Check sheet for the modelled part. Datum: model origin and axes. Units: mm. A direction names the side the tool comes from. Round coordinates to 2 decimals unless told otherwise and drop trailing zeros. Use one line per item in the form item = value. Start each with the question number.
Autodesk Inventor part; units mm, degrees
ref_plane "YZ Plane" through (0, 0, 0) normal (1, 0, 0) x (0, 1, 0)
ref_plane "XZ Plane" through (0, 0, 0) normal (0, 1, 0) x (-1, 0, 0)
ref_plane "XY Plane" through (0, 0, 0) normal (0, 0, 1) x (1, 0, 0)
sketch "Skizze1" plane through (0, 0, 0) normal (0, 1, 0) x (-1, 0, 0)
  line L0 (77.2474, 30) -> (-16.7526, 30)
  line L1 (-16.7526, 30) -> (-16.7526, -30)
  line L2 (-16.7526, -30) -> (77.2474, -30)
  line L3 (77.2474, -30) -> (77.2474, 30)
  line L4 (-35.5526, 0) -> (96.0474, 0)
  point P0 (0, 0)
  dimension "d0" = 30
  dimension "d1" = 60
  dimension "d2" = 94
extrude "Extrusion1" add sketch "Skizze1" along normal blind 10
sketch "Skizze4" plane through (0, 10, 0) normal (0, 1, 0) x (1, 0, 0)
  circle A0 centre (-14.4974, -15.75) radius 2
  circle A1 centre (-14.4974, 15.75) radius 2
  circle A2 centre (-45.9974, -15.75) radius 2
  circle A3 centre (-45.9974, 15.75) radius 2
  line L0 (35.5526, 0) -> (-96.0474, 0)
  line L1 (16.7526, -30) -> (16.7526, 30)
  line L2 (-77.2474, 30) -> (-77.2474, -30)
  point P0 (0, 0)
  dimension "d21" = 4
  dimension "d22" = 15.75
  dimension "d23" = 15.75
  dimension "d26" = 15.75
  dimension "d27" = 15.75
  dimension "d30" = 4
  dimension "d31" = 4
  dimension "d32" = 4
  dimension "d127" = 31.5
  dimension "d128" = 31.5
  dimension "d129" = 31.25
  dimension "d130" = 31.25
extrude "Extrusion4" cut sketch "Skizze4" against normal blind 10
sketch "Skizze5" plane through (0, 10, 0) normal (0, 1, 0) x (1, 0, 0)
  line L0 (-6.9974, -24) -> (-21.9974, -24)
  line L1 (-21.9974, -24) -> (-21.9974, 24)
  line L2 (-21.9974, 24) -> (-6.9974, 24)
  line L3 (-6.9974, 24) -> (-6.9974, -24)
  line L4 (-38.4974, 24) -> (-53.4974, 24)
  line L5 (-53.4974, 24) -> (-53.4974, -24)
  line L6 (-53.4974, -24) -> (-38.4974, -24)
  line L7 (-38.4974, -24) -> (-38.4974, 24)
  line L8 (35.5526, 0) -> (-96.0474, 0)
  line L9 (16.7526, -30) -> (16.7526, 30)
  line L10 (-77.2474, 30) -> (-77.2474, -30)
  point P0 (0, 0)
  dimension "d35" = 15
  dimension "d36" = 48
  dimension "d37" = 24
  dimension "d38" = 23.75
  dimension "d39" = 15
  dimension "d189" = 16.5
extrude "Extrusion5" cut sketch "Skizze5" against normal blind 1
sketch "Skizze6" plane through (0, 9, 0) normal (0, 1, 0) x (1, 0, 0)
  circle A0 centre (-14.4974, -15.75) radius 3.6
  circle A1 centre (-14.4974, 15.75) radius 3.6
  circle A2 centre (-45.9974, -15.75) radius 3.6
  circle A3 centre (-45.9974, 15.75) radius 3.6
  circle A4 centre (-45.9974, 15.75) radius 2
  circle A5 centre (-45.9974, -15.75) radius 2
  circle A6 centre (-14.4974, 15.75) radius 2
  circle A7 centre (-14.4974, -15.75) radius 2
  circle A8 centre (-3.2474, -15.75) radius 3.6
  circle A9 centre (-3.2474, 15.75) radius 3.6
  circle A10 centre (-45.9974, -15.75) radius 3.6
  circle A11 centre (-53.2474, 15.75) radius 3.6
  circle A12 centre (-53.2474, 15.75) radius 2
  circle A13 centre (-45.9974, -15.75) radius 2
  circle A14 centre (-3.2474, 15.75) radius 2
  circle A15 centre (-3.2474, -15.75) radius 2
  circle A16 centre (-3.2474, -15.75) radius 3.6
  circle A17 centre (-3.2474, 15.75) radius 3.6
  circle A18 centre (-45.9974, -15.75) radius 3.6
  circle A19 centre (-53.2474, 15.75) radius 3.6
  circle A20 centre (-53.2474, 15.75) radius 2
  circle A21 centre (-45.9974, -15.75) radius 2
  circle A22 centre (-3.2474, 15.75) radius 2
  circle A23 centre (-3.2474, -15.75) radius 2
  circle A24 centre (-3.2474, -15.75) radius 3.6
  circle A25 centre (-3.2474, 15.75) radius 3.6
  circle A26 centre (-53.2474, -15.75) radius 3.6
  circle A27 centre (-53.2474, 15.75) radius 3.6
  circle A28 centre (-53.2474, 15.75) radius 2
  circle A29 centre (-53.2474, -15.75) radius 2
  circle A30 centre (-3.2474, 15.75) radius 2
  circle A31 centre (-3.2474, -15.75) radius 2
  line L0 (-77.2474, 30) -> (-77.2474, -30)
  point P0 (0, 0)
  point P1 (0, 0)
  point P2 (0, 0)
  point P3 (0, 0)
  point P4 (-45.7474, 16.7182)
  point P5 (-45.7474, 14.7818)
  point P6 (-45.7474, -14.7818)
  point P7 (-45.7474, -16.7182)
  point P8 (-10.7474, 14.7818)
  point P9 (-10.7474, 16.7182)
  point P10 (-10.7474, -16.7182)
  point P11 (-10.7474, -14.7818)
  dimension "d43" = 7.2
  dimension "d44" = 7.2
  dimension "d45" = 7.2
  dimension "d46" = 7.2
  dimension "d79" = 7.2
  dimension "d80" = 7.2
  dimension "d81" = 7.2
  dimension "d82" = 7.2
  dimension "d83" = 7.2
  dimension "d84" = 7.2
  dimension "d85" = 7.2
  dimension "d86" = 7.2
  dimension "d87" = 7.2
  dimension "d88" = 7.2
  dimension "d89" = 7.2
  dimension "d90" = 7.2
  dimension "d142" = 31.25
  dimension "d143" = 31.25
extrude "Extrusion6" cut sketch "Skizze6" against normal blind 3 contours A0 | A1 | A2 | A3 | A4 | A5 | A6 | A7
sketch "Skizze8" plane through (0, 9, 0) normal (0, 1, 0) x (1, 0, 0)
  circle A0 centre (-14.4974, -5.0565) radius 1.5
  circle A1 centre (-14.4974, 4.9435) radius 1.5
  circle A2 centre (-45.9974, -5.0565) radius 1.5
  circle A3 centre (-45.9974, 4.9435) radius 1.5
  line L0 (-77.2474, 30) -> (-77.2474, -30)
  line L1 (16.7526, -30) -> (16.7526, 30)
  point P0 (0, 0)
  dimension "d56" = 10
  dimension "d57" = 10
  dimension "d58" = 31.25
  dimension "d59" = 31.25
  dimension "d62" = 3
  dimension "d63" = 3
  dimension "d64" = 3
  dimension "d65" = 3
  dimension "d146" = 31.25
extrude "Extrusion7" cut sketch "Skizze8" against normal blind 10
chamfer "Fase1" distance 0.5 angle 45 4 edges at (-47.9974, 6, 15.75) (-47.9974, 6, -15.75) (-16.4974, 6, -15.75) (-16.4974, 6, 15.75)
sketch "Skizze9" plane through (0, 0, 0) normal (0, -1, 0) x (1, 0, 0)
  line L0 (-6.9974, -24) -> (-21.9974, -24)
  line L1 (-21.9974, -24) -> (-21.9974, 24)
  line L2 (-21.9974, 24) -> (-6.9974, 24)
  line L3 (-6.9974, 24) -> (-6.9974, -24)
  line L4 (-38.4974, 24) -> (-53.4974, 24)
  line L5 (-53.4974, 24) -> (-53.4974, -24)
  line L6 (-53.4974, -24) -> (-38.4974, -24)
  line L7 (-38.4974, -24) -> (-38.4974, 24)
  line L8 (34.7526, 0) -> (-91.2474, 0)
  line L9 (16.7526, 30) -> (16.7526, -30)
  line L10 (-77.2474, -30) -> (-77.2474, 30)
  point P0 (0, 0)
  point P1 (0, 0)
  dimension "d71" = 15
  dimension "d72" = 48
  dimension "d73" = 24
  dimension "d75" = 15
  dimension "d144" = 23.75
  dimension "d145" = 23.75
extrude "Extrusion8" cut sketch "Skizze9" against normal blind 1
sketch "Skizze10" plane through (0, 0, 0) normal (0, -1, 0) x (1, 0, 0)
  circle A0 centre (-14.4974, -15.75) radius 3.6
  circle A1 centre (-14.4974, 15.75) radius 3.6
  circle A2 centre (-45.9974, -15.75) radius 3.6
  circle A3 centre (-45.9974, 15.75) radius 3.6
  circle A4 centre (-45.9974, 15.75) radius 2
  circle A5 centre (-45.9974, -15.75) radius 2
  circle A6 centre (-14.4974, 15.75) radius 2
  circle A7 centre (-14.4974, -15.75) radius 2
  circle A8 centre (-3.2474, -15.75) radius 3.6
  circle A9 centre (-3.2474, 15.75) radius 3.6
  circle A10 centre (-45.9974, -15.75) radius 3.6
  circle A11 centre (-53.2474, 15.75) radius 3.6
  circle A12 centre (-53.2474, 15.75) radius 2
  circle A13 centre (-45.9974, -15.75) radius 2
  circle A14 centre (-3.2474, 15.75) radius 2
  circle A15 centre (-3.2474, -15.75) radius 2
  circle A16 centre (-3.2474, -15.75) radius 3.6
  circle A17 centre (-3.2474, 15.75) radius 3.6
  circle A18 centre (-53.2474, -15.75) radius 3.6
  circle A19 centre (-53.2474, 15.75) radius 3.6
  circle A20 centre (-53.2474, 15.75) radius 2
  circle A21 centre (-53.2474, -15.75) radius 2
  circle A22 centre (-3.2474, 15.75) radius 2
  circle A23 centre (-3.2474, -15.75) radius 2
  circle A24 centre (-3.2474, -15.75) radius 3.6
  circle A25 centre (-3.2474, 15.75) radius 3.6
  circle A26 centre (-53.2474, -15.75) radius 3.6
  circle A27 centre (-53.2474, 15.75) radius 3.6
  circle A28 centre (-53.2474, 15.75) radius 2
  circle A29 centre (-53.2474, -15.75) radius 2
  circle A30 centre (-3.2474, 15.75) radius 2
  circle A31 centre (-3.2474, -15.75) radius 2
  line L0 (-77.2474, -30) -> (-77.2474, 30)
  line L1 (16.7526, 30) -> (16.7526, -30)
  point P0 (0, 0)
  point P1 (0, 0)
  point P2 (0, 0)
  point P3 (0, 0)
  point P4 (0, 0)
  dimension "d91" = 7.2
  dimension "d92" = 7.2
  dimension "d93" = 7.2
  dimension "d94" = 7.2
  dimension "d95" = 7.2
  dimension "d96" = 7.2
  dimension "d97" = 7.2
  dimension "d98" = 7.2
  dimension "d99" = 7.2
  dimension "d100" = 7.2
  dimension "d101" = 7.2
  dimension "d102" = 7.2
  dimension "d103" = 7.2
  dimension "d104" = 7.2
  dimension "d105" = 7.2
  dimension "d106" = 7.2
  dimension "d147" = 31.25
  dimension "d148" = 31.25
  dimension "d149" = 31.25
  dimension "d150" = 31.25
  dimension "d151" = 31.25
extrude "Extrusion9" cut sketch "Skizze10" against normal blind 4 contours A0 | A1 | A2 | A3 | A4 | A5 | A6 | A7
sketch "Skizze12" plane through (0, 10, 0) normal (0, 1, 0) x (1, 0, 0)
  circle A0 centre (-71.2474, -15) radius 1.5
  circle A1 centre (-71.2474, 15) radius 1.5
  circle A2 centre (10.7526, 15) radius 1.5
  circle A3 centre (10.7526, -15) radius 1.5
  line L0 (-77.2474, 30) -> (-77.2474, -30)
  line L1 (16.7526, -30) -> (16.7526, 30)
  point P0 (0, 0)
  dimension "d121" = 3
  dimension "d122" = 3
  dimension "d123" = 3
  dimension "d124" = 3
  dimension "d131" = 82
  dimension "d132" = 82
  dimension "d138" = 6
  dimension "d139" = 6
extrude "Extrusion11" cut sketch "Skizze12" against normal blind 60
sketch "Skizze15" plane through (-77.2474, 0, -30) normal (-1, 0, 0) x (0, 0, 1)
  circle A0 centre (38, 5) radius 1.15
  circle A1 centre (22, 5) radius 1.15
  line L0 (30, 12) -> (30, -2)
  line L1 (0, 10) -> (60, 10)
  point P0 (30, 0)
  dimension "d158" = 8
  dimension "d159" = 8
  dimension "d160" = 5
  dimension "d163" = 2.3
  dimension "d164" = 2.3
extrude "Extrusion13" cut sketch "Skizze15" against normal blind 10
chamfer "Fase2" distance 2 angle 45 2 edges at (-77.2474, 5, 6.85) (-77.2474, 5, -9.15)
sketch "Skizze16" plane through (16.7526, 0, 30) normal (1, 0, 0) x (0, 0, -1)
  circle A0 centre (38, 5) radius 1.15
  circle A1 centre (22, 5) radius 1.15
  line L0 (0, 10) -> (60, 10)
  line L1 (30, -2) -> (30, 12)
  point P0 (30, 0)
  dimension "d168" = 5
  dimension "d169" = 5
  dimension "d170" = 8
  dimension "d171" = 8
  dimension "d172" = 2.3
  dimension "d173" = 2.3
extrude "Extrusion14" cut sketch "Skizze16" against normal blind 10
chamfer "Fase3" distance 2 angle 45 2 edges at (16.7526, 5, 9.15) (16.7526, 5, -6.85)
sketch "Skizze17" plane through (0, 0, 0) normal (0, -1, 0) x (1, 0, 0)
  line L0 (16.7526, 30) -> (11.7526, 30)
  line L1 (16.7526, 29) -> (11.7526, 30)
  line L2 (16.7526, 29) -> (16.7526, 30)
  line L3 (16.7526, -30) -> (11.7526, -30)
  line L4 (16.7526, -29) -> (11.7526, -30)
  line L5 (16.7526, -29) -> (16.7526, -30)
  line L6 (-77.2474, -30) -> (-72.2474, -30)
  line L7 (-77.2474, -30) -> (-77.2474, -29)
  line L8 (-77.2474, -29) -> (-72.2474, -30)
  line L9 (-77.2474, 30) -> (-72.2474, 30)
  line L10 (-77.2474, 30) -> (-77.2474, 29)
  line L11 (-77.2474, 29) -> (-72.2474, 30)
  point P0 (0, 0)
  dimension "d179" = 1
  dimension "d180" = 5
  dimension "d181" = 5
  dimension "d182" = 1
  dimension "d183" = 1
  dimension "d184" = 5
  dimension "d185" = 5
  dimension "d186" = 1
extrude "Extrusion15" cut sketch "Skizze17" against normal blind 10
properties part number "guidingplate"
1. Depth check by flat-ended pin: pin 1 (6 mm diameter, centred on y = 6.5, z = -8, fed in from +X); pin 2 (2 mm diameter, centred on x = -47.5, z = -15, fed in from +Y); pin 3 (0.7 mm diameter, centred on y = 4.5, z = -8, fed in from -X); pin 4 (6 mm diameter, centred on x = -45, z = 17, fed in from +Y). Enter the tip coordinate at first touch or a pass-through.
2. Tool access check on faces 1 (the face through (-71.3, 5.97, -7.38)), 2 (the face through (-48.854, 2.479, -17.941)), 3 (the face through (-46, 9, 0)). Record the directions out of +Z, -Z, +X, -X, +Y, -Y that give a thin tool (end or side, any length) a straight path to the whole face; none if there is none.
3. Mould release check, pull along Y, two halves, no side actions. Record for faces 4 (the face through (6.753, 5, 8)), 5 (the face through (-13, 4, 14)), 6 (the face through (-15, 9, 0)): +Y half, -Y half, draft (parallel to the pull), parting line (faces both ways), or undercut.
4. Scan lines: probe 1 along X at (y, z) = (6.25, 15); probe 2 along X at (y, z) = (1.75, 12.5); probe 3 along Y at (x, z) = (-53, 15.5). Record each from-to range of solid material in increasing order.
Returned:
q1.pin_1 = 16.75
q1.pin_2 = 6
q1.pin_3 = -67.25
q1.pin_4 = 9
q2.face_1 = -X
q2.face_2 = -Y
q2.face_3 = +Y
q3.face_4 = undercut
q3.face_5 = -Y half
q3.face_6 = +Y half
q4.probe_1 = -77.25 to -72.75, -69.75 to -49.52, -42.48 to -18.02, -10.98 to 9.25, 12.25 to 16.75
q4.probe_2 = -77.25 to -47.55, -44.45 to -16.05, -12.95 to 16.75
q4.probe_3 = 1 to 9
